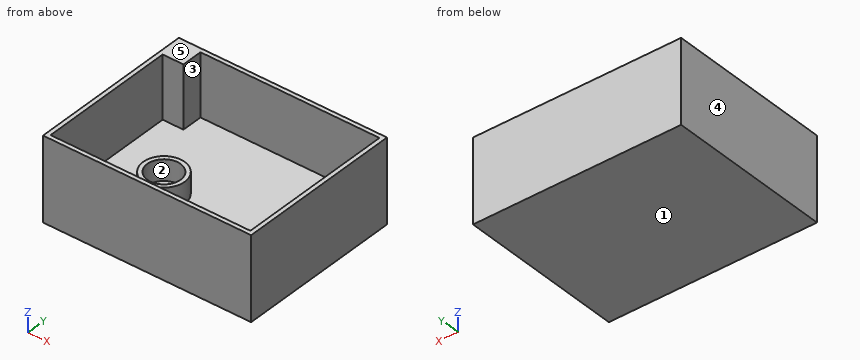
from build123d import *

# Parameters (mm, degrees)
F0_W     = 50
F0_H     = 40
F1_DEPTH = 20
F2_W     = 48
F2_H     = 38
F3_DEPTH = 15
F4_W     = 5
F4_H     = 5
F5_DEPTH = 15
F6_R     = 5
F6_R_2   = 4
F7_DEPTH = 5


with BuildPart() as f1:
    # F0 (on Top) → F1 (new body)
    with BuildSketch(Plane.XY):
        Rectangle(F0_W, F0_H)
    extrude(amount=F1_DEPTH)

    # F2 (on face) → F3 (cut)
    with BuildSketch(Plane.XY.offset(20)):
        Rectangle(F2_W, F2_H)
    extrude(amount=-F3_DEPTH, mode=Mode.SUBTRACT)

    # F4 (on face) → F5 (join)
    with BuildSketch(Plane.XY.offset(5)):
        with Locations((-21.5, 16.5)):
            Rectangle(F4_W, F4_H)
    extrude(amount=F5_DEPTH)

    # F6 (on face) → F7 (join)
    with BuildSketch(Plane.XY.offset(5)):
        with Locations((-9, -4)):
            Circle(F6_R)
        with Locations((-9, -4)):
            Circle(F6_R_2, mode=Mode.SUBTRACT)
    extrude(amount=F7_DEPTH)


solid = f1.part
Verification items for the finished model (mm, model axes). Face numbers are marked on the shaded views. A direction names the side the tool comes from. Give positions to 0.01 mm unless a question says otherwise; leave off trailing zeros. Loops run counter-clockwise (first coordinate to the right, second up) from the corner with the lowest first, then second, coordinate; pieces in that order, holes last. Notation, with made-up numbers: (-22, 70.5) - (-8, 70.5) arc R24 cw to (-8, 105.5) - close; hole circle Ø11 at (8.25, 81). An arc over 180 degrees is marked (long way). Write each question's results on one line, items separated by ' | '.
1) Depth check by flat-ended pin: P1, Ø5, axis at x = 19.5, y = -8.5, coming from the +Z side. Enter the tip coordinate at first touch or a pass-through.
Solution:
P1: z = 5
2) Sectioned sample at A-A on z = 7.75. Record the boundary of the cut face in (x, y), plus the area to 3 significant figures.
Solution:
outline: (-25, -20) - (25, -20) - (25, 20) - (-25, 20) - close; circle Ø10 at (-9, -4); hole (-24, -19) - (24, -19) - (24, 19) - (-19, 19) - (-19, 14) - (-24, 14) - close; hole circle Ø8 at (-9, -4) | area: 229 mm2
3) Sectioned sample at D-D on z = 14.5. Record the boundary of the cut face in (x, y), plus the area to 3 significant figures.
Solution:
outline: (-25, -20) - (25, -20) - (25, 20) - (-25, 20) - close; hole (-24, -19) - (24, -19) - (24, 19) - (-19, 19) - (-19, 14) - (-24, 14) - close | area: 201 mm2
4) Material ranges on L1, parallel to Y at x = -9, z = 8.5; L2, parallel to Y at x = 19, z = 12.5; L3, parallel to X at y = 7, z = 5.25, recorded low to high. Write a range as from..to.
Solution:
L1: -20..-19, -9..-8, 0..1, 19..20 | L2: -20..-19, 19..20 | L3: -25..-24, 24..25
5) Tool access check on the marked faces 1 and 2. Record the directions out of +Z, -Z, +X, -X, +Y, -Y that give a thin tool (end or side, any length) a straight path to the whole face; none if there is none.
Solution:
face 1: -Z, +X, -X, +Y, -Y | face 2: +Z
6) Sectioned sample at B-B on x = -9. Record the boundary of the cut face in (y, z), plus the area to 3 significant figures.
Solution:
outline: (-20, 0) - (20, 0) - (20, 20) - (19, 20) - (19, 5) - (1, 5) - (1, 10) - (0, 10) - (0, 5) - (-8, 5) - (-8, 10) - (-9, 10) - (-9, 5) - (-19, 5) - (-19, 20) - (-20, 20) - close | area: 240 mm2
7) Mould release check, pull along X, two halves, no side actions. Record for the marked faces 3, 4 and 5: pulls with the +X half, pulls with the -X half, needs draft (parallel to the pull), parting line crosses it, or undercut.
Solution:
face 3: undercut | face 4: pulls with the -X half | face 5: needs draft
8) Sectioned sample at C-C on y = 15. Record the boundary of the cut face in (x, z).
Solution:
outline: (-25, 0) - (25, 0) - (25, 20) - (24, 20) - (24, 5) - (-19, 5) - (-19, 20) - (-25, 20) - close
